Geometry check sheet. Reference: the model listing, model coordinates, mm. A direction names the side the tool comes from. Give positions to 0.01 mm unless a question says otherwise; leave off trailing zeros. Write each loop counter-clockwise with the first axis right and the second up, starting at its lowest first coordinate (ties: lowest second). Pieces come first, ordered by that corner, then holes. Notation, with made-up numbers: (30.5, 33.5) - (49.5, 33.5) arc R16 cw to (49.5, 55.5) - close; hole circle Ø11 at (71, 29.5). An arc over 180 degrees is marked (long way). Use a Markdown table: item, result.
Autodesk Inventor part; units mm, degrees
ref_plane "YZ Plane" through (0, 0, 0) normal (1, 0, 0) x (0, 1, 0)
ref_plane "XZ Plane" through (0, 0, 0) normal (0, 1, 0) x (-1, 0, 0)
ref_plane "XY Plane" through (0, 0, 0) normal (0, 0, 1) x (1, 0, 0)
sketch "Sketch1" plane through (0, 0, 0) normal (0, 0, 1) x (1, 0, 0)
  line L0 (0, 0) -> (50, 0)
  line L1 (50, 0) -> (50, 18.4)
  line L2 (50, 18.4) -> (0, 18.4)
  line L3 (0, 18.4) -> (0, 0)
  line L4 (0, 12.4) -> (16, 12.4)
  line L5 (16, 12.4) -> (16, 6)
  line L6 (16, 6) -> (0, 6)
  line L7 (0, 6) -> (0, 12.4)
  line L8 (58.8783, 9.2) -> (-7.6234, 9.2)
  point P0 (0, 6)
  dimension "d0" = 50
  dimension "d1" = 18.4
  dimension "d11" = 16
  dimension "d13" = 18.4
  dimension "d14" = 6.4
  dimension "d15" = 6.4
extrude "Extrusion1" add sketch "Sketch1" along normal blind 8 contours L3 L6 L5 L8 L1 L0 | L8 L5 L4 L3 L2 L1
fillet "Fillet1" radius 4 4 edges at (0, 3, 8) (0, 3, 0) (0, 15.4, 8) (0, 15.4, 0)
sketch "Sketch3" plane through (50, 0, 0) normal (0, -1, 0) x (1, 0, 0)
  circle A0 centre (-46, 4) radius 2.05
  line L0 (-46, 8) -> (0, 8)
  arc A1 (-46, 8) -> (-46, 0) centre (-46, 4) ccw
  circle A2 centre (-39, 2.6) radius 1.6
  line L1 (-46, 0) -> (0, 0)
  circle A3 centre (-46, 4) radius 4
  line L2 (-44.7623, 7.8037) -> (-30, 3)
  line L3 (-30, 3) -> (-8, 3)
  line L4 (-8, 3) -> (0, 8)
  line L5 (0, 0) -> (0, 8)
  line L6 (-7.1396, 0) -> (0, 4.4623)
  line L7 (0, 4.4623) -> (-1.59, 7.0063)
  point P0 (-50, 0)
  point P1 (-50, 4)
  point P2 (-50, 4)
  point P3 (-50, 4)
  point P4 (-4, 5.5)
  dimension "d23" = 8
  dimension "d17" = 4.1
  dimension "d18" = 4
  dimension "d19" = 4
  dimension "d20" = 3.2
  dimension "d21" = 2.6
  dimension "d22" = 11
  dimension "d24" = 20
  dimension "d25" = 8
  dimension "d26" = 5
  dimension "d27" = 3
extrude "Extrusion3" cut sketch "Sketch3" against normal blind 20 contours A0 | L0 L4 L3 L2 A3 | L5 L7 L4 | L5 L1 L6 | A2
properties part number "Lever"
1) Section check C-C on y = 8.5. Record the boundary of the cut face in (x, z).
Working result:
| item | result |
|---|---|
| outline | (16, 0) - (42.86, 0) - (50, 4.46) - (48.41, 7.01) - (42, 3) - (20, 3) - (16, 4.3) - close |
2) Section check D-D on x = 33. Record the boundary of the cut face in (y, z), then the cut area to 3 significant figures.
Working result:
| item | result |
|---|---|
| outline | (0, 0) - (18.4, 0) - (18.4, 3) - (0, 3) - close |
| area | 55.2 mm² |
3) Material ranges on L1, parallel to Y at x = 5, z = 2; L2, parallel to Z at x = 4, y = 2; L3, parallel to X at y = 1.25, z = 1.25, recorded low to high. Write a range as from..to.
Working result:
| item | result |
|---|---|
| L1 | y = 0..6, 12.4..18.4 |
| L2 | z = 0..1.95, 6.05..8 |
| L3 | x = 1.1..10.14, 11.86..44.86 |
4) Depth check by flat-ended pin: P1, Ø1.5, axis at x = 24.5, y = 11.5, coming from the +Z side; P2, Ø1.3, axis at y = 9, z = 2, coming from the -X side; P3, Ø1.5, axis at x = 9, z = 4.5, coming from the -Y side; P4, Ø10, axis at x = 43, y = 13, coming from the +Z side. Enter the tip coordinate at first touch or a pass-through.
Working result:
| item | result |
|---|---|
| P1 | stops at z = 3 |
| P2 | stops at x = 16 |
| P3 | stops at y = 0 |
| P4 | stops at z = 6.75 |
5) Mould release check, pull along X, two halves, no side actions. Record for faces 4 (the flat face through (8, 12.4, 3)), 5 (the cylindrical face through (2.373, 15.358, 2.753)), 6 (the cylindrical face through (1.141, 2.958, 1.203)): pulls with the +X half, pulls with the -X half, needs draft (parallel to the pull), parting line crosses it, or undercut.
Working result:
| item | result |
|---|---|
| face 4 | needs draft |
| face 5 | undercut |
| face 6 | pulls with the -X half |
6) Set-up check for faces 1 (the cylindrical face through (1.141, 15.358, 1.203)), 2 (the flat face through (45.2, 9.1, 5)), 3 (the flat face through (8, 6, 3)): record each of +Z, -Z, +X, -X, +Y, -Y from which the full face is reachable in a straight line by a thin tool's end or side.
Working result:
| item | result |
|---|---|
| face 1 | -Z, -X, +Y, -Y |
| face 2 | +Z, +Y, -Y |
| face 3 | +Z, -Z, -X |
7) Section check A-A on y = 3.5. Count the separate pieces of the cut face and the enclosed holes in it, then the cut area to 3 significant figures.
Working result:
| item | result |
|---|---|
| separate pieces | 1 |
| enclosed holes | 2 |
| area | 185 mm² |
8) Section check B-B on x = 11. Record the boundary of the cut face in (y, z), then the cut area to 3 significant figures.
Working result:
| item | result |
|---|---|
| outline | (0, 0) - (6, 0) - (6, 1) - (0, 1) - close; (0, 4.2) - (6, 4.2) - (6, 5.93) - (0, 5.93) - close; (12.4, 0) - (18.4, 0) - (18.4, 1) - (12.4, 1) - close; (12.4, 4.2) - (18.4, 4.2) - (18.4, 5.93) - (12.4, 5.93) - close |
| area | 32.7 mm² |
